Can you work these out from the drawing? Everything is in mm from the part's minimum corner. A direction names the side the tool comes from. Give positions to 0.01 mm unless a question says otherwise; leave off trailing zeros. Write each loop counter-clockwise with the first axis right and the second up, starting at its lowest first coordinate (ties: lowest second). Pieces come first, ordered by that corner, then holes. Notation, with made-up numbers: (67.25, 38.25) -> (76.25, 38.25) arc R28 cw to (76.25, 75.25) -> close; hole circle Ø3 at (-12.5, -36). An arc over 180 degrees is marked (long way). Return JSON: item names as keys, results as strings.
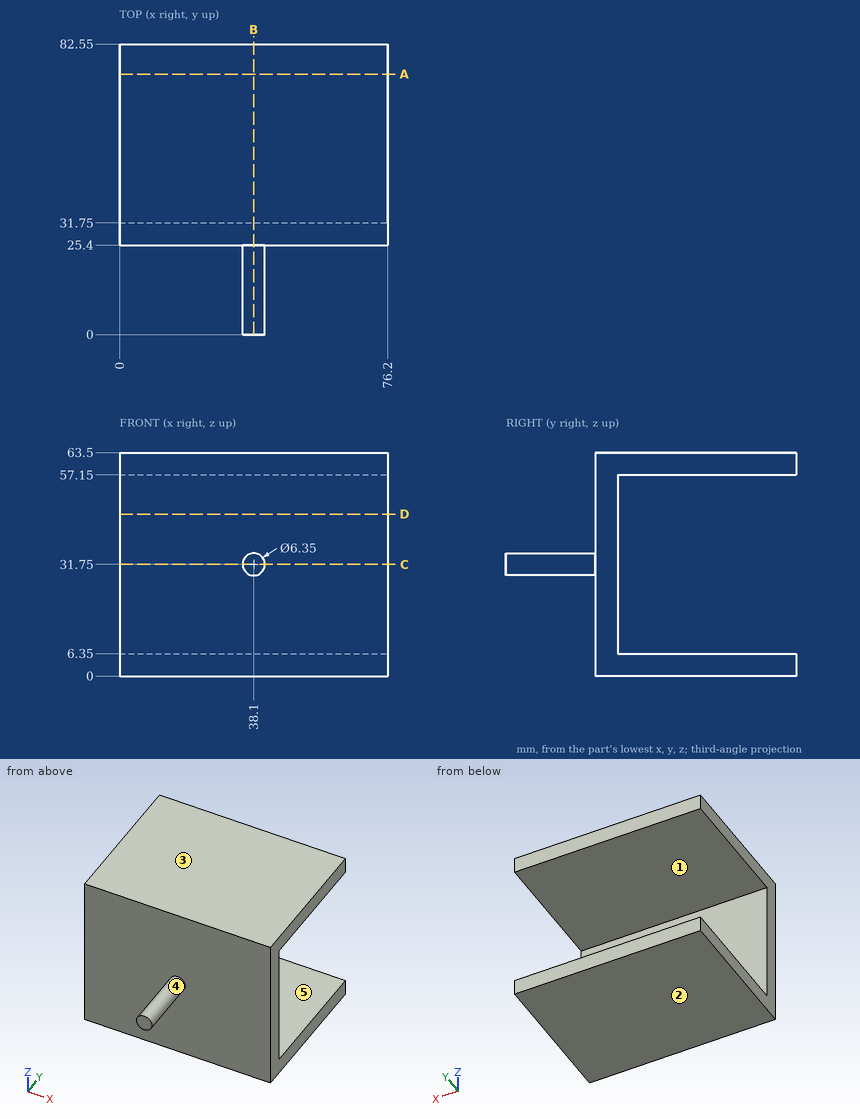
1. If I drill on line 1 (Z direction, x = 60, y = 72); line 2 (Y direction, x = 9, z = 42.5); line 3 (Y direction, x = 58, z = 5.5), over which ranges is the centre line in solid material (lowest first)? Write a range as [from, to].
Taken from the geometry:
{"line 1": "z = [0, 6.35], [57.15, 63.5]", "line 2": "y = [25.4, 31.75]", "line 3": "y = [25.4, 82.55]"}
2. Suppose I cut it at A-A, the plane y = 74. List the corners of the cut face in (x, z) for me.
Taken from the geometry:
{"outline": "(0, 0) -> (76.2, 0) -> (76.2, 6.35) -> (0, 6.35) -> close; (0, 57.15) -> (76.2, 57.15) -> (76.2, 63.5) -> (0, 63.5) -> close"}
3. Suppose I cut it at D-D, the plane z = 46. List the corners of the cut face in (x, y) for me, and give its area (3 significant figures).
Taken from the geometry:
{"outline": "(0, 25.4) -> (76.2, 25.4) -> (76.2, 31.75) -> (0, 31.75) -> close", "area": "484 mm²"}
4. Suppose I cut it at C-C, the plane z = 31.75. List the corners of the cut face in (x, y) for me (3 decimals).
Taken from the geometry:
{"outline": "(0, 25.4) -> (34.925, 25.4) -> (34.925, 0) -> (41.275, 0) -> (41.275, 25.4) -> (76.2, 25.4) -> (76.2, 31.75) -> (0, 31.75) -> close"}
5. If we mould it in two halves opening along Z, with no side actions, what happens to the marked faces 3, 4 and 5? For each: released by +Z, released by -Z, zero draft, split by the parting line, or undercut.
Taken from the geometry:
{"face 3": "released by +Z", "face 4": "split by the parting line", "face 5": "undercut"}
6. Which directions (+Z, -Z, +X, -X, +Y, -Y) give clear straight access to the entire face, cutting with the end or side of a thin tool? Please do the marked faces 1 and 2.
Taken from the geometry:
{"face 1": "+X, -X, +Y", "face 2": "-Z, +X, -X, +Y, -Y"}
7. For pin 1 Ø5 at (x, z) = (61.5, 52.5) entering from -Y; pin 2 Ø5 at (x, z) = (43.5, 32.5) entering from +Y; pin 3 Ø1.5 at (y, z) = (20, 28.5) entering from +X, each with a flat end and sliding along its axis, tell me the tip position at first contact or that it passes through.
Taken from the geometry:
{"pin 1": "stops at y = 25.4", "pin 2": "stops at y = 31.75", "pin 3": "stops at x = 40.06"}
8. Suppose I cut it at B-B, the plane x = 38.1. List the corners of the cut face in (y, z) for me (3 decimals).
Taken from the geometry:
{"outline": "(0, 28.575) -> (25.4, 28.575) -> (25.4, 0) -> (82.55, 0) -> (82.55, 6.35) -> (31.75, 6.35) -> (31.75, 57.15) -> (82.55, 57.15) -> (82.55, 63.5) -> (25.4, 63.5) -> (25.4, 34.925) -> (0, 34.925) -> close"}
